The figure shows three views and two pictorial views of one solid part (mm, origin at its lowest corner). Answer the questions. Give positions to 0.01 mm unless a question says otherwise; leave off trailing zeros. Loops run counter-clockwise (first coordinate to the right, second up) from the corner with the lowest first, then second, coordinate; pieces in that order, holes last. Notation, with made-up numbers: M 76.25,6.5 L 110.25,6.5 A24 cw 110.25,45.5 Z; hole C 70.25,-1 d10. An arc over 180 degrees is marked long. One line per item, written item: value. Start each with the question number.
Q1. A cutting plane is placed at A-A, the plane z = 28.5. Determine the outline of the cut face in (x, y), and give its area (3 significant figures).
Q2. Consider L1, parallel to X at y = 31, z = 7.5; L2, parallel to Z at x = 14, y = 30.5; L3, parallel to Z at x = 34.5, y = 35. Determine where each line is inside the solid, lowest interval first.
Q3. Flat-ended cylindrical pins translate along their axes: pin 1 (1 mm diameter, centred on y = 36, z = 12.5, fed in from -X); pin 2 (4 mm diameter, centred on x = 33.5, y = 41, fed in from +Z); pin 3 (6 mm diameter, centred on y = 35, z = 8, fed in from -X). Find the tip coordinate at first contact, or state that the pin passes through.
Q4. A cutting plane is placed at D-D, the plane y = 16.5. Determine the outline of the cut face in (x, z).
Q5. A cutting plane is placed at C-C, the plane y = 3.5. Determine the outline of the cut face in (x, z), and give its area (3 significant figures).
Q6. A cutting plane is placed at B-B, the plane x = 22. Determine the outline of the cut face in (y, z).
Q7. The mould has two halves that part along X. Classify the marked faces 1 and 2: +X half, -X half, draft (parallel to the pull), parting line (faces both ways), or undercut.
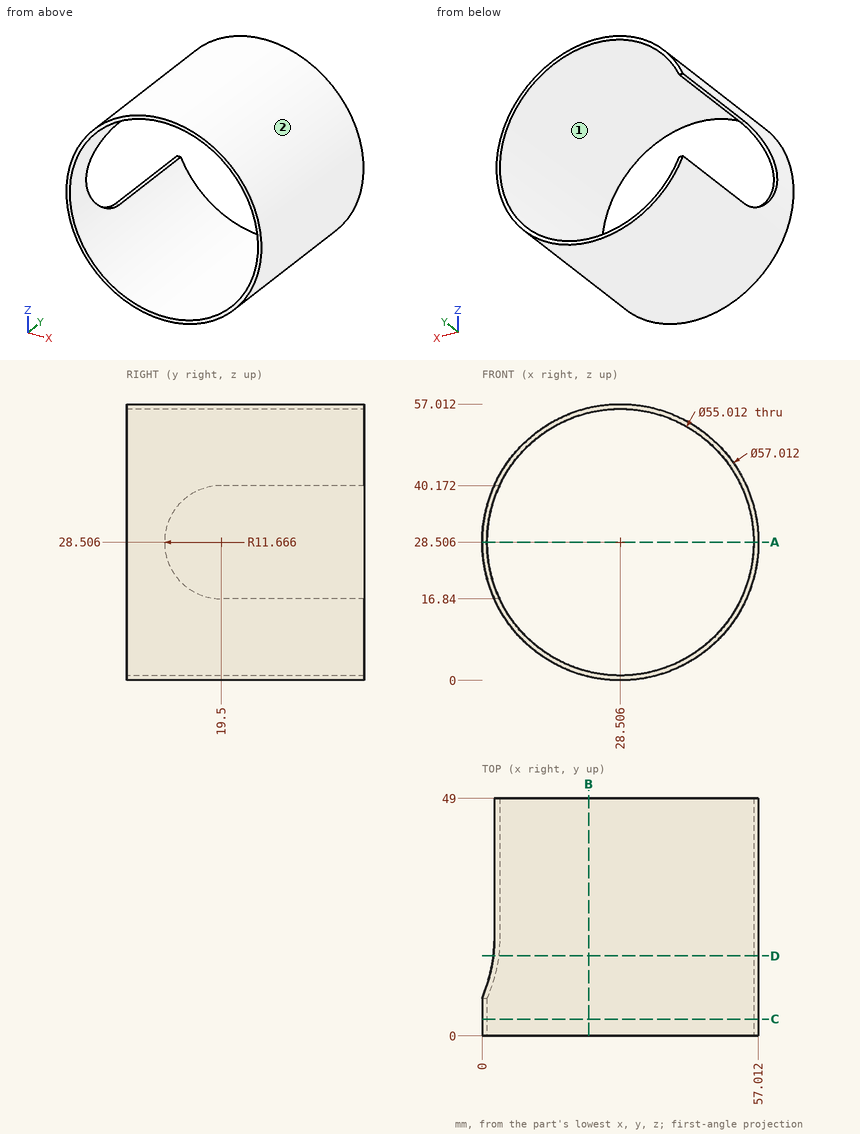
Answer block:
1. outline: M 0,0 L 1,0 L 1,7.83 L 0,7.83 Z; M 56.01,0 L 57.01,0 L 57.01,49 L 56.01,49 Z
1. area: 56.8 mm^2
2. L1: 9.24 to 10.75, 46.26 to 47.78
2. L2: 3.97 to 5.14, 51.88 to 53.05
2. L3: 0.64 to 1.66, 55.35 to 56.37
3. pin 1: x = 4.59
3. pin 2: z = 56.85
3. pin 3: x = 6.01
4. outline: M 2.32,17.23 A28.51 ccw long 2.32,39.78 L 3.42,39.78 A27.51 cw long 3.42,17.23 Z
5. outline: C 28.51,28.51 d57.01; hole C 28.51,28.51 d55.01
5. area: 176 mm^2
6. outline: M 0,0.75 L 49,0.75 L 49,1.78 L 0,1.78 Z; M 0,55.23 L 49,55.23 L 49,56.26 L 0,56.26 Z
7. face 1: undercut
7. face 2: parting line
